The model under review builds one solid part; all positions refer to its coordinate system, in mm. Coordinates: 2 decimals unless noted, no trailing zeros. Loops run counter-clockwise (first coordinate to the right, second up) from the corner with the lowest first, then second, coordinate; pieces in that order, holes last. Notation, with made-up numbers: M 59,32.25 L 111,32.25 A11 cw 111,41.25 Z; hole C -11.5,13 d9. An arc over 180 degrees is marked long. Return JSON: item names as keys, results as strings.
```python
from build123d import *

# Parameters (mm, degrees)
SKETCH_W     = 53
SKETCH_H     = 31.8
PAD_DEPTH    = 3
SKETCH001_R  = 5.85
POCKET_DEPTH = 3.001


with BuildPart() as part:
    # Sketch → Pad (new body)
    with BuildSketch(Plane.XY):
        with Locations((36.5, 25.9)):
            Rectangle(SKETCH_W, SKETCH_H)
    extrude(amount=PAD_DEPTH)

    # Sketch001 → Pocket (cut, through all)
    with BuildSketch(Plane.XY):
        with Locations((36, 25.9)):
            Circle(SKETCH001_R)
    extrude(amount=POCKET_DEPTH, mode=Mode.SUBTRACT)


solid = part.part
```
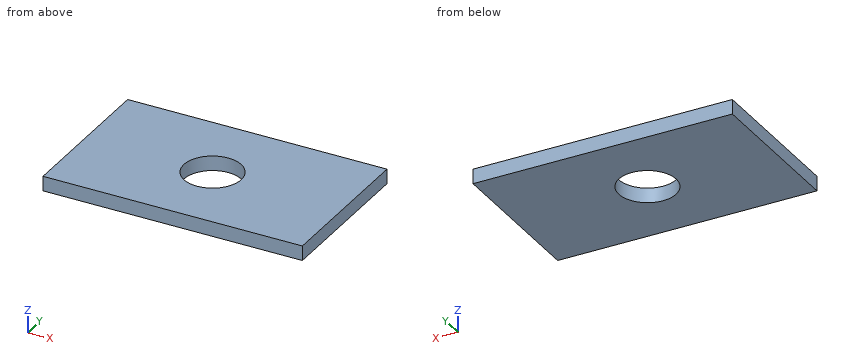
1. Add section B-B on y = 25.9. Give the boundary of the cut face in (x, z), plus the area to 3 significant figures.
Check values:
{"outline": "M 10,0 L 30.15,0 L 30.15,3 L 10,3 Z; M 41.85,0 L 63,0 L 63,3 L 41.85,3 Z", "area": "124 mm²"}
2. Add section A-A on x = 36. Give the boundary of the cut face in (y, z), plus the area to 3 significant figures.
Check values:
{"outline": "M 10,0 L 20.05,0 L 20.05,3 L 10,3 Z; M 31.75,0 L 41.8,0 L 41.8,3 L 31.75,3 Z", "area": "60.3 mm²"}
3. To check wall thickness, follow line 1 (Y direction, x = 36, z = 1.3); line 2 (X direction, y = 25.9, z = 1.25); line 3 (Y direction, x = 39.5, z = 0.7). State the ranges of each line that lie inside material, in increasing order.
Check values:
{"line 1": "10 to 20.05, 31.75 to 41.8", "line 2": "10 to 30.15, 41.85 to 63", "line 3": "10 to 21.21, 30.59 to 41.8"}
4. Add section C-C on z = 1.45. Give the boundary of the cut face in (x, y), plus the area to 3 significant figures.
Check values:
{"outline": "M 10,10 L 63,10 L 63,41.8 L 10,41.8 Z; hole C 36,25.9 d11.7", "area": "1,580 mm²"}
5. Insertion check: pin 1 Ø3 at (x, y) = (18, 35.5) entering from -Z. The pin has a flat end and moves straight along its axis. Give the tip position at first contact, or say it passes through.
Check values:
{"pin 1": "z = 0"}
